Part model, mm, in its own coordinate system. A direction names the side the tool comes from. Round coordinates to 2 decimals unless told otherwise and drop trailing zeros. Write each loop counter-clockwise with the first axis right and the second up, starting at its lowest first coordinate (ties: lowest second). Pieces come first, ordered by that corner, then holes. Notation, with made-up numbers: M 70.5,0 L 99.5,0 A22 cw 99.5,34 Z; hole C -27,53.5 d7. An arc over 180 degrees is marked long. One line per question, with ' | ' between items. Start each with the question number.
1) Saw through at B-B (y = 21.1). List the corners of the cut face in (x, z), plus the area to 3 significant figures.
2) Saw through at A-A (x = 0). List the corners of the cut face in (y, z).
3) Mould opens along X. For faces 3 (the face through (-11.38, 3.73, 12.32)), 4 (the face through (-2.84, 8.31, 12.32)), 5 (the face through (0, 5, 7)) say: pulls with the +X half, pulls with the -X half, needs draft (parallel to the pull), parting line crosses it, or undercut.
4) Wall check: probe 1 along Z at (x, y) = (-4.5, 3.5); probe 2 along X at (y, z) = (-18.5, 15.75); probe 3 along Y at (x, z) = (3.5, 17.25). Give the ranges that are in metal, low to high. Write a range as [from, to].
5) Saw through at C-C (z = 18). List the corners of the cut face in (x, y).
6) Drop flat-ended pins along their axis: pin 1 Ø4 at (x, z) = (-10.5, 11.5) entering from +Y; pin 2 Ø1 at (y, z) = (13, 10) entering from +X; pin 3 Ø3 at (x, z) = (4, 19.5) entering from -Y; pin 4 Ø2 at (x, y) = (2.5, 3.5) entering from -Z. Give the stop position or say it passes through.
7) Tool access for faces 1 (the face through (0, 4, 9.5)), 2 (the face through (0.512, -0.007, 12.325)): list every direction of +Z, -Z, +X, -X, +Y, -Y with a clear straight run to the whole face (end or side of a thin tool).
8) Saw through at D-D (y = -18.5). List the corners of the cut face in (x, z).
```python
from build123d import *

# Parameters (mm, degrees)
SKETCH_R          = 13.1
PAD_DEPTH         = 25
SKETCH001_W       = 2
SKETCH001_H       = 5.5
POCKET_DEPTH      = 22.001
POCKET_DEPTH_BACK = 22.001


with BuildPart() as part:
    # Sketch → Pad (new body)
    with BuildSketch(Plane.XY):
        with BuildLine():
            ThreePointArc((17, -25.79726), (0, 0), (-17, -25.79726))
            ThreePointArc((-20.216216, -27.177822), (-17.917827, -28.095649), (-17, -25.79726))
            ThreePointArc((-14.206112, -1.701596), (-21.412232, -13.448634), (-20.216216, -27.177822))
            ThreePointArc((-14.206112, -1.701596), (-11.372558, 3.815069), (-13.288911, 9.713392))
            ThreePointArc((13.288911, 9.713392), (0, 38.6), (-13.288911, 9.713392))
            ThreePointArc((13.288911, 9.713392), (11.372558, 3.815069), (14.206112, -1.701596))
            ThreePointArc((20.216216, -27.177822), (21.412232, -13.448634), (14.206112, -1.701596))
            ThreePointArc((17, -25.79726), (17.917827, -28.095649), (20.216216, -27.177822))
        make_face()
        with Locations((0, 21.1)):
            Circle(SKETCH_R, mode=Mode.SUBTRACT)
    extrude(amount=PAD_DEPTH)

    # Sketch001 → Pocket (cut, two sides)
    with BuildSketch(Plane.YZ) as pocket_sk:
        with Locations((4, 6.75)):
            Rectangle(SKETCH001_W, SKETCH001_H)
        with Locations((4, 18.25)):
            Rectangle(SKETCH001_W, SKETCH001_H)
    extrude(amount=-POCKET_DEPTH, mode=Mode.SUBTRACT)
    extrude(pocket_sk.sketch, amount=POCKET_DEPTH_BACK, mode=Mode.SUBTRACT)


solid = part.part
```
Answer key:
1) outline: M -17.5,0 L -13.1,0 L -13.1,25 L -17.5,25 Z; M 13.1,0 L 17.5,0 L 17.5,25 L 13.1,25 Z | area: 220 mm2
2) outline: M 0,0 L 8,0 L 8,25 L 0,25 Z; M 34.2,0 L 38.6,0 L 38.6,25 L 34.2,25 Z; hole M 3,4 L 5,4 L 5,9.5 L 3,9.5 Z; hole M 3,15.5 L 5,15.5 L 5,21 L 3,21 Z
3) face 3: pulls with the -X half | face 4: undercut | face 5: needs draft
4) probe 1: z = [0, 4], [9.5, 15.5], [21, 25] | probe 2: x = [-22, -18.5], [18.5, 22] | probe 3: y = [-0.33, 3], [5, 8.48], [33.72, 38.25]
5) outline: M -20.22,-27.18 A1.75 ccw -17,-25.8 A18.5 cw long 17,-25.8 A1.75 ccw 20.22,-27.18 A22 ccw 14.21,-1.7 A8.07 cw 11.48,3 L -11.48,3 A8.07 cw -14.21,-1.7 A22 ccw Z; M -13.29,9.71 A8.07 cw -11.36,5 L 11.36,5 A8.07 cw 13.29,9.71 A17.5 ccw long Z; hole C 0,21.1 d26.2
6) pin 1: stops at y = 36.4 | pin 2: stops at x = 15.76 | pin 3: stops at y = -0.84 | pin 4: stops at z = 0
7) face 1: +X, -X | face 2: +Z, -Z
8) outline: M -22,0 L -18.5,0 L -18.5,25 L -22,25 Z; M 18.5,0 L 22,0 L 22,25 L 18.5,25 Z
